Could you check a few things on this model? Use its own coordinates, in mm. A direction names the side the tool comes from. Round coordinates to 2 decimals unless told otherwise and drop trailing zeros. Loops run counter-clockwise (first coordinate to the right, second up) from the corner with the lowest first, then second, coordinate; pieces in that order, holes last. Notation, with made-up numbers: (-2, -3.75) -> (57, -3.75) arc R26 ccw to (57, 28.25) -> close; hole circle Ø3 at (-36, 81). An arc over 180 degrees is marked (long way). Write each question's results on one line, items separated by ' | '.
from build123d import *

# Parameters (mm, degrees)
F0_R     = 5.25
F0_R_2   = 3.25
F0_R_3   = 1.75
F1_DEPTH = 7
F2_R     = 6.99999
F3_DEPTH = 5
F4_DEPTH = 0.2
F5_SIZE  = 0.5
F6_R     = 2.75
F6_R_2   = 1.75
F7_DEPTH = 0.5


# Not quite as in the source:
# - a fillet or chamfer is up to 0.001 mm smaller than in the source, because OpenCascade refuses the exact size
# - a feature names something its author has since deleted; it is built from what else it names


with BuildPart() as f1:
    # F0 (on Top) → F1 (new body)
    with BuildSketch(Plane.XY):
        with BuildLine():
            Line((10.5, 11), (-10.5, 11))
            ThreePointArc((-10.5, 11), (-18.2781745931, 7.7781745931), (-21.5, 0))
            ThreePointArc((-21.5, 0), (-18.2781745931, -7.7781745931), (-10.5, -11))
            Line((-10.5, -11), (10.5, -11))
            ThreePointArc((10.5, -11), (18.2781745931, -7.7781745931), (21.5, 0))
            ThreePointArc((21.5, 0), (18.2781745931, 7.7781745931), (10.5, 11))
        make_face()
        with Locations((-12.25, 0)):
            Circle(F0_R, mode=Mode.SUBTRACT)
        with Locations((12.25, 0)):
            Circle(F0_R, mode=Mode.SUBTRACT)
        with Locations((-12.25, 0)):
            Circle(F0_R)
        with Locations((-12.25, 0)):
            Circle(F0_R_2, mode=Mode.SUBTRACT)
        with Locations((12.25, 0)):
            Circle(F0_R)
        with Locations((12.25, 0)):
            Circle(F0_R_2, mode=Mode.SUBTRACT)
        with Locations((12.25, 0)):
            Circle(F0_R_2)
        with Locations((12.25, 0)):
            Circle(F0_R_3, mode=Mode.SUBTRACT)
        with Locations((-12.25, 0)):
            Circle(F0_R_2)
        with Locations((-12.25, 0)):
            Circle(F0_R_3, mode=Mode.SUBTRACT)
        with Locations((-12.25, 0)):
            Circle(F0_R_3)
        with Locations((12.25, 0)):
            Circle(F0_R_3)
    extrude(amount=F1_DEPTH)

    # F2 (radius 7 in the source; OpenCascade refuses exactly that, so slightly less here)
    f2_edges = [f1.edges().sort_by_distance(p)[0] for p in [
        (0, 11, 7),
    ]]
    fillet(f2_edges, radius=F2_R)

    # F0 (on Top) → F3 (join)
    with BuildSketch(Plane.XY):
        with Locations((12.25, 0)):
            Circle(F0_R_2)
        with Locations((12.25, 0)):
            Circle(F0_R_3, mode=Mode.SUBTRACT)
        with Locations((-12.25, 0)):
            Circle(F0_R_2)
        with Locations((-12.25, 0)):
            Circle(F0_R_3, mode=Mode.SUBTRACT)
    extrude(amount=-F3_DEPTH)

    # F0 (on Top) → F4 (cut)
    with BuildSketch(Plane.XY):
        with Locations((-12.25, 0)):
            Circle(F0_R)
        with Locations((-12.25, 0)):
            Circle(F0_R_2, mode=Mode.SUBTRACT)
        with Locations((12.25, 0)):
            Circle(F0_R)
        with Locations((12.25, 0)):
            Circle(F0_R_2, mode=Mode.SUBTRACT)
    extrude(amount=F4_DEPTH, mode=Mode.SUBTRACT)

    # F5
    f5_edges = [f1.edges().sort_by_distance(p)[0] for p in [
        (-15.5, 0, 0.2),
        (9, 0, 0.2),
    ]]
    chamfer(f5_edges, length=F5_SIZE)

    # F6 (on face) → F7 (cut)
    with BuildSketch(Plane(origin=(0, 0, -5), x_dir=(1, 0, 0), z_dir=(0, 0, -1))):
        with Locations((-12.25, 0)):
            Circle(F6_R)
        with Locations((-12.25, 0)):
            Circle(F6_R_2, mode=Mode.SUBTRACT)
        with Locations((12.25, 0)):
            Circle(F6_R)
    extrude(amount=-F7_DEPTH, mode=Mode.SUBTRACT)


solid = f1.part
1) For faces 4 (the flat face through (-12, 0, 0)), 5 (the cylindrical face through (-0.1, 9, 4.9)), which set-ups out of +Z, -Z, +X, -X, +Y, -Y let a thin tool reach every point of the face, with its end or its side?
Model answer:
face 4: -Z | face 5: +Z, +X, -X, +Y
2) I want a section at A-A, the plane z = -3.5. Write out the boundary of the cut face in (x, y), plus the area to 3 significant figures.
Model answer:
outline: circle Ø6.5 at (-12.25, 0); circle Ø6.5 at (12.25, 0); hole circle Ø3.5 at (-12.25, 0); hole circle Ø3.5 at (12.25, 0) | area: 47.1 mm2
3) I need wall thicknesses on line 1 (Y direction, x = -12.25, z = -4.75); line 2 (Y direction, x = -12.25, z = -1.8); line 3 (Y direction, x = -12.25, z = 0.15). Which ranges of each line are inside material? Lowest first, please.
Model answer:
line 1: y = -3.25 to -2.75, 2.75 to 3.25 | line 2: y = -3.25 to -1.75, 1.75 to 3.25 | line 3: y = -10.86 to -5.25, -3.7 to 3.7, 5.25 to 10.86
4) If we mould it in two halves opening along Y, with no side actions, what happens to faces 1 (the flat face through (13, 3, -5)), 2 (the cylindrical face through (0.1, -9, 4.9)), 3 (the flat face through (12, 2, -4.5))? For each: released by +Y, released by -Y, zero draft, split by the parting line, or undercut.
Model answer:
face 1: zero draft | face 2: released by -Y | face 3: undercut
5) I'm going to push flat-ended pins straight in: pin 1 (4 mm diameter, centred on y = -2.5, z = -2.5, fed in from -X); pin 2 (3 mm diameter, centred on x = 12.25, y = 0, fed in from -Z); pin 3 (1.5 mm diameter, centred on x = -12.5, y = 4.5, fed in from +Z). Where does each tip first touch, or does it pass through?
Model answer:
pin 1: stops at x = -15.46 | pin 2: stops at z = 0 | pin 3: stops at z = 7
